Geometry check sheet. Reference: the model listing, model coordinates, mm. Coordinates: 2 decimals unless noted, no trailing zeros. Write each loop counter-clockwise with the first axis right and the second up, starting at its lowest first coordinate (ties: lowest second). Pieces come first, ordered by that corner, then holes. Notation, with made-up numbers: (51, -4) -> (86, -4) arc R27 cw to (86, 33) -> close; hole circle Ø2 at (-23, 84). An arc over 180 degrees is marked (long way). One line per question, with ' | ' between items.
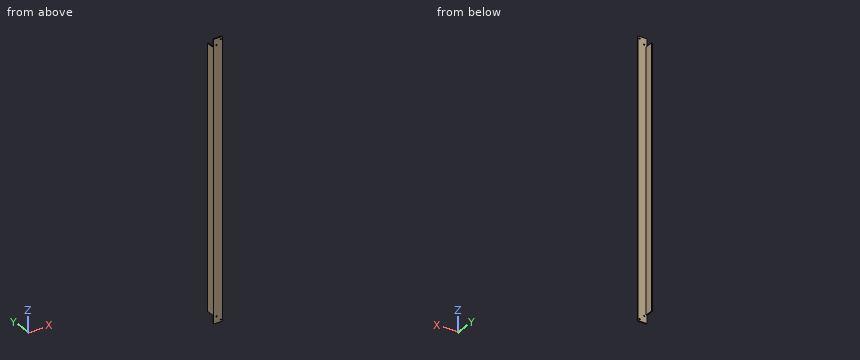
from build123d import *

# Parameters (mm, degrees)
BOSS_EXTRU_1_DEPTH      = 614
ESQUISSE2_W             = 18
ESQUISSE2_H             = 18
ENL_V_MAT_EXTRU_1_DEPTH = 3
ESQUISSE6_R             = 1.4
ENL_V_MAT_EXTRU_5_DEPTH = 3


with BuildPart() as part:
    # Esquisse1 → Boss.-Extru.1 (new body)
    with BuildSketch(Plane.XY):
        Polygon((0, 0), (20, 0), (20, 2), (2, 2), (2, 20), (0, 20), align=None)
    extrude(amount=BOSS_EXTRU_1_DEPTH)

    # Esquisse2 → Enlèv. mat.-Extru.1 (cut, through all)
    with BuildSketch(Plane(origin=(2, 0, 0), x_dir=(0, 0, -1), z_dir=(1, 0, 0))):
        with Locations((-605, 11)):
            Rectangle(ESQUISSE2_W, ESQUISSE2_H)
        with Locations((-9, 11)):
            Rectangle(ESQUISSE2_W, ESQUISSE2_H)
    extrude(amount=-ENL_V_MAT_EXTRU_1_DEPTH, mode=Mode.SUBTRACT)

    # Esquisse6 → Enlèv. mat.-Extru.5 (cut, through all)
    with BuildSketch(Plane(origin=(0, 2, 0), x_dir=(1, 0, 0), z_dir=(0, 1, 0))):
        with Locations((6.48, -599.52)):
            Circle(ESQUISSE6_R)
        with Locations((6.48, -14.48)):
            Circle(ESQUISSE6_R)
        with Locations((16.48, -609.52)):
            Circle(ESQUISSE6_R)
        with Locations((16.48, -4.48)):
            Circle(ESQUISSE6_R)
    extrude(amount=-ENL_V_MAT_EXTRU_5_DEPTH, mode=Mode.SUBTRACT)


solid = part.part
1. Cross-section at A-A on z = 513. Record the boundary of the cut face in (x, y).
Worked answers:
outline: (0, 0) -> (20, 0) -> (20, 2) -> (2, 2) -> (2, 20) -> (0, 20) -> close
2. Cross-section at B-B on y = 15.5. Record the boundary of the cut face in (x, z), and give its area (3 significant figures).
Worked answers:
outline: (0, 18) -> (2, 18) -> (2, 596) -> (0, 596) -> close | area: 1,160 mm²
3. Material ranges on line 1 (Z direction, x = 6.48, y = 0.9); line 2 (X direction, y = 0.5, z = 609.52); line 3 (Y direction, x = 7, z = 176), recorded low to high. Write a range as from..to.
Worked answers:
line 1: 0..13.08, 15.88..598.12, 600.92..614 | line 2: 0..15.08, 17.88..20 | line 3: 0..2
4. Go/stop test with flat-tipped pins: P1, Ø1, axis at x = 5.5, z = 459.5, coming from the +Y side; P2, Ø1.5, axis at y = 8, z = 300, coming from the +X side; P3, Ø12, axis at x = 16.5, y = 11.5, coming from the +Z side; P4, Ø0.6, axis at x = 1, y = 9.5, coming from the +Z side. Record where each tip stops, or that it passes through.
Worked answers:
P1: y = 2 | P2: x = 2 | P3: through | P4: z = 596
